from build123d import *

# Parameters (mm, degrees)
BOSS_EXTRUDE1_DEPTH         = 4.7625
F_6_CLEARANCE_HOLE1_D       = 4.3053
F_3_4_0_75_DIAMETER_HOLE1_D = 19.05


with BuildPart() as part:
    # Sketch1 → Boss-Extrude1 (new body)
    with BuildSketch(Plane.XY):
        with BuildLine():
            Line((-133.0325, 57.658), (-133.0325, 50.8))
            ThreePointArc((-133.0325, 50.8), (-134.520397552, 47.207897552), (-138.1125, 45.72))
            Line((-138.1125, 45.72), (-140.716, 45.72))
            Line((-140.716, 45.72), (-140.716, 17.018))
            Line((-140.716, 17.018), (-28.956, 17.018))
            Line((-28.956, 17.018), (-28.956, 47.498))
            Line((-28.956, 47.498), (-39.116, 57.658))
            Line((-39.116, 57.658), (-133.0325, 57.658))
        make_face()
    extrude(amount=BOSS_EXTRUDE1_DEPTH)

    # #6 Clearance Hole1 (through all)
    with Locations(Plane.XY.offset(4.7625)):
        with Locations((-133.35, 30.1625), (-35.56, 43.688)):
            Hole(F_6_CLEARANCE_HOLE1_D / 2)

    # 3/4 (0.75) Diameter Hole1 (through all)
    with Locations(Plane.XY.offset(4.7625)):
        with Locations((-112.7125, 33.528), (-52.3875, 33.528)):
            Hole(F_3_4_0_75_DIAMETER_HOLE1_D / 2)


solid = part.part
Geometry check sheet. Reference: the model listing, model coordinates, mm. A direction names the side the tool comes from. Round coordinates to 2 decimals unless told otherwise and drop trailing zeros. Loops run counter-clockwise (first coordinate to the right, second up) from the corner with the lowest first, then second, coordinate; pieces in that order, holes last.
Item 1: Mould release check, pull along X, two halves, no side actions. Record for faces 1 (the flat face through (-28.956, 32, 2)), 2 (the cylindrical face through (-131.2, 30.3, 2.3)), 3 (the flat face through (-86, 38, 4.762)): pulls with the +X half, pulls with the -X half, needs draft (parallel to the pull), parting line crosses it, or undercut.
Item 2: Access from +Z, -Z, +X, -X, +Y, -Y to the whole of each face (thin tool, end or side, straight path). Record for faces 4 (the flat face through (-133.032, 54, 2)), 5 (the flat face through (-85, 57.658, 2)).
Item 3: Cross-section at B-B on x = -35.56. Record the boundary of the cut face in (y, z), then the cut area to 3 significant figures.
Item 4: Cross-section at C-C on z = 2.1. Count the separate pieces of the cut face and the enclosed holes in it, then the cut area to 3 significant figures.
Item 5: Cross-section at D-D on y = 34.5. Record the boundary of the cut face in (x, z).
Item 6: Cross-section at A-A on y = 26. Record the boundary of the cut face in (x, z), then the cut area to 3 significant figures.
Item 7: Gauge pin test, flat ends, axial feed: pin 1 (1.4 mm diameter, centred on y = 54, z = 3.5, fed in from -X); pin 2 (17 mm diameter, centred on x = -112.71, y = 33.53, fed in from +Z); pin 3 (1.3 mm diameter, centred on x = -139, z = 1.5, fed in from +Y). Record the tip position at first contact, or that the pin passes through.
Item 8: Thickness scan on line 1 (X direction, y = 33, z = 2.45); line 2 (Y direction, x = -35.56, z = 3.85); line 3 (Y direction, x = -51, z = 1.7). Record the ranges inside material, lowest first.
Answer sheet:
1. face 1: pulls with the +X half
1. face 2: undercut
1. face 3: needs draft
2. face 4: +Z, -Z, -X, +Y
2. face 5: +Z, -Z, +X, -X, +Y
3. outline: (17.02, 0) - (41.54, 0) - (41.54, 4.76) - (17.02, 4.76) - close; (45.84, 0) - (54.1, 0) - (54.1, 4.76) - (45.84, 4.76) - close
3. area: 156 mm2
4. separate pieces: 1
4. enclosed holes: 4
4. area: 3,800 mm2
5. outline: (-140.72, 0) - (-122.19, 0) - (-122.19, 4.76) - (-140.72, 4.76) - close; (-103.24, 0) - (-61.86, 0) - (-61.86, 4.76) - (-103.24, 4.76) - close; (-42.91, 0) - (-28.96, 0) - (-28.96, 4.76) - (-42.91, 4.76) - close
6. outline: (-140.72, 0) - (-118.55, 0) - (-118.55, 4.76) - (-140.72, 4.76) - close; (-106.88, 0) - (-58.22, 0) - (-58.22, 4.76) - (-106.88, 4.76) - close; (-46.55, 0) - (-28.96, 0) - (-28.96, 4.76) - (-46.55, 4.76) - close
6. area: 421 mm2
7. pin 1: stops at x = -133.03
7. pin 2: passes through
7. pin 3: stops at y = 45.72
8. line 1: x = -140.72 to -122.22, -103.2 to -61.9, -42.88 to -28.96
8. line 2: y = 17.02 to 41.54, 45.84 to 54.1
8. line 3: y = 17.02 to 24.1, 42.95 to 57.66
